Read the model definition and answer for the solid it produces. Units are mm, in the model's axes. Coordinates: 2 decimals unless noted, no trailing zeros. Order: outer loops, then holes, each group sorted by start corner. A loop starts at its lowest first (then second) coordinate and runs counter-clockwise, first axis right, second up. Notation, with made-up numbers: (6, -7.75) - (19, -7.75) arc R19 ccw to (19, 13.25) - close; hole circle Ø1 at (47, 5.5). An arc over 180 degrees is marked (long way). Use one line per item in the form item = value.
```python
from build123d import *

# Parameters (mm, degrees)
BOSS_EXTRUDE1_DEPTH = 76.2
SKETCH13_R          = 7.5
CUT_EXTRUDE1_DEPTH  = 269


with BuildPart() as part:
    # Sketch1 → Boss-Extrude1 (new body)
    with BuildSketch(Plane(origin=(0, 0, 0), x_dir=(1, 0, 0), z_dir=(0, 1, 0))):
        with BuildLine():
            ThreePointArc((235.021699517, -237.381311512), (0, -253), (-235.021699517, -237.381311512))
            Line((-235.021699517, -237.381311512), (-235.021699517, -252.381311512))
            ThreePointArc((-235.021699517, -252.381311512), (0, -268), (235.021699517, -252.381311512))
            Line((235.021699517, -252.381311512), (235.021699517, -237.381311512))
        make_face()
    extrude(amount=BOSS_EXTRUDE1_DEPTH)

    # Sketch13 → Cut-Extrude1 (cut, through all)
    with BuildSketch(Plane.XY):
        with Locations((0, 38.1)):
            Circle(SKETCH13_R)
    extrude(amount=CUT_EXTRUDE1_DEPTH, mode=Mode.SUBTRACT)


solid = part.part
```
(1) Section B-B, the plane y = 38.1 is taken. Write down the section's boundary in (x, z), then the cut area to 3 significant figures.
Answer list:
outline = (-235.02, 237.38) arc R1776.05 cw to (-7.5, 252.98) - (-7.5, 267.98) arc R1776.05 ccw to (-235.02, 252.38) - close; (7.5, 252.98) arc R1776.05 cw to (235.02, 237.38) - (235.02, 252.38) arc R1776.05 ccw to (7.5, 267.98) - close
area = 6,830 mm2
(2) Section D-D, the plane y = 5.5 is taken. Write down the section's boundary in (x, z), then the cut area to 3 significant figures.
Answer list:
outline = (-235.02, 237.38) arc R1776.05 cw to (235.02, 237.38) - (235.02, 252.38) arc R1776.05 ccw to (-235.02, 252.38) - close
area = 7,050 mm2
(3) The mould has two halves that part along X. Classify faces 1 (the cylindrical face through (-3.3, 46.033, 267.997)), 2 (the flat face through (-3, 76.2, 256)), 3 (the cylindrical face through (-0.976, 45.536, 260.387)): +X half, -X half, draft (parallel to the pull), parting line (faces both ways), or undercut.
Answer list:
face_1 = parting line
face_2 = draft
face_3 = undercut
(4) Section A-A, the plane x = 0 is taken. Write down the section's boundary in (y, z), then the cut area to 3 significant figures.
Answer list:
outline = (0, 253) - (30.6, 253) - (30.6, 268) - (0, 268) - close; (45.6, 253) - (76.2, 253) - (76.2, 268) - (45.6, 268) - close
area = 918 mm2
(5) Given pin 1 Ø1 at (x, z) = (-171.5, 247.5) entering from -Y; pin 2 Ø1 at (x, y) = (32, 61.5) entering from -Z, each flat-ended and moving along its own axis, determine where each tip first touches the part or whether it passes through.
Answer list:
pin_1 = 0
pin_2 = 252.7
(6) Straight lines are drawn through the part: L1, parallel to Y at x = 0, z = 263; L2, parallel to Z at x = -109, y = 27; L3, parallel to Z at x = 112, y = 41.5. For each, find the intervals that lie inside material, in ascending order.
Answer list:
L1 = 0 to 30.6, 45.6 to 76.2
L2 = 249.65 to 264.65
L3 = 249.47 to 264.47
